from build123d import *

# Parameters (mm, degrees)
SKETCH_1_R      = 5
EXTRUDE_1_DEPTH = 3


with BuildPart() as part:
    # 草图1 → 凸台-拉伸1 (new body)
    with BuildSketch(Plane(origin=(0, 0, 0), x_dir=(1, 0, 0), z_dir=(0, 1, 0))):
        with BuildLine():
            Line((-1.5, -14.924811557), (-1.5, -10))
            Line((-1.5, -10), (1.5, -10))
            Line((1.5, -10), (1.5, -14.924811557))
            ThreePointArc((1.5, -14.924811557), (15, 0), (1.5, 14.924811557))
            Line((1.5, 14.924811557), (1.5, 10))
            Line((1.5, 10), (-1.5, 10))
            Line((-1.5, 10), (-1.5, 14.924811557))
            ThreePointArc((-1.5, 14.924811557), (-15, 0), (-1.5, -14.924811557))
        make_face()
        with Locations(Location((0, 0, 0), (0, 0, 270))):
            Circle(SKETCH_1_R, mode=Mode.SUBTRACT)
    extrude(amount=EXTRUDE_1_DEPTH)


solid = part.part
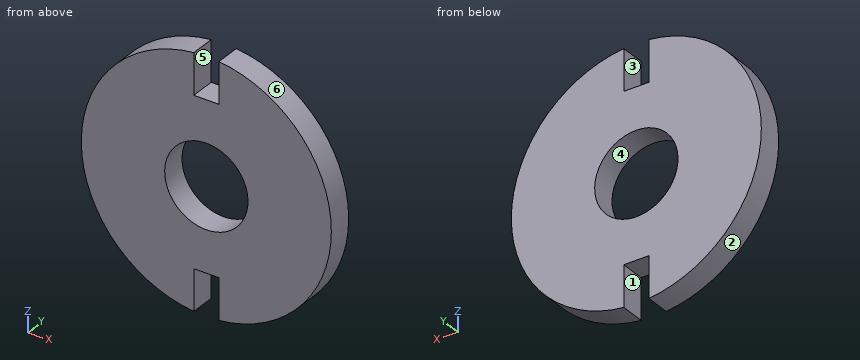
Model file for the job. Use its own axes, mm. Face numbers are marked on the shaded views. A direction names the side the tool comes from. Give positions to 0.01 mm unless a question says otherwise; leave off trailing zeros. Loops run counter-clockwise (first coordinate to the right, second up) from the corner with the lowest first, then second, coordinate; pieces in that order, holes last.
1) Saw through at C-C (y = 1.05). Write the cut outline in (x, z).
2) Pull direction Z, two halves, no side cores. Call the marked faces 4, 5 and 6: +Z half, -Z half, draft (parallel to the pull), parting line (faces both ways), or undercut.
3) Tool access for the marked faces 1, 2 and 3: list every direction of +Z, -Z, +X, -X, +Y, -Y with a clear straight run to the whole face (end or side of a thin tool).
4) Saw through at B-B (x = 0). Write the cut outline in (y, z), plus the area to 3 significant figures.
5) Saw through at D-D (x = -6). Write the cut outline in (y, z), plus the area to 3 significant figures.
6) Wall check: line 1 (X direction, y = 2.1, z = 0); line 2 (X direction, y = 1.9, z = 3.25); line 3 (Z direction, x = 1.75, y = 0.6). Give the ranges that are in metal, low to high.
7) Saw through at A-A (z = 0). Write the cut outline in (x, y), plus the area to 3 significant figures.
8) Flat gauge pins, fed straight in: pin 1 Ø1.5 at (y, z) = (1, -13.5) entering from +X; pin 2 Ø6 at (x, z) = (0, 0) entering from +Y; pin 3 Ø3 at (x, z) = (3, 8.5) entering from -Y; pin 4 Ø1.5 at (y, z) = (1, 12.5) entering from -X. Where does each tip first touch, or does it go through?
Answer block:
1. outline: (-1.5, -14.92) - (-1.5, -10) - (1.5, -10) - (1.5, -14.92) arc R15 ccw to (1.5, 14.92) - (1.5, 10) - (-1.5, 10) - (-1.5, 14.92) arc R15 ccw to start; hole circle Ø10 at (0, 0)
2. face 4: undercut
2. face 5: draft
2. face 6: parting line
3. face 1: -Z, +Y, -Y
3. face 2: -X, +Y, -Y
3. face 3: +Z, +Y, -Y
4. outline: (0, -10) - (3, -10) - (3, -5) - (0, -5) - close; (0, 5) - (3, 5) - (3, 10) - (0, 10) - close
4. area: 30.0 mm2
5. outline: (0, -13.75) - (3, -13.75) - (3, 13.75) - (0, 13.75) - close
5. area: 82.5 mm2
6. line 1: x = -15 to -5, 5 to 15
6. line 2: x = -14.64 to -3.8, 3.8 to 14.64
6. line 3: z = -14.9 to -4.68, 4.68 to 14.9
7. outline: (-15, 0) - (-5, 0) - (-5, 3) - (-15, 3) - close; (5, 0) - (15, 0) - (15, 3) - (5, 3) - close
7. area: 60.0 mm2
8. pin 1: stops at x = 7.9
8. pin 2: passes through
8. pin 3: stops at y = 0
8. pin 4: stops at x = -9.32
